from build123d import *

# Parameters (mm, degrees)
SKETCH_1_R           = 82.5
EXTRUDE_1_DEPTH      = 22.5
EXTRUDE_1_DEPTH_BACK = 22.5
SKETCH_4_R           = 67.5
CUT_EXTRUDE_1_DEPTH  = 4
SKETCH_5_R           = 52
CUT_EXTRUDE_2_DEPTH  = 48
CUT_EXTRUDE_3_DEPTH  = 2


with BuildPart() as part:
    # Sketch 1 → Extrude 1 (new body, two sides)
    with BuildSketch(Plane.XY) as extrude_1_sk:
        Circle(SKETCH_1_R)
    extrude(amount=EXTRUDE_1_DEPTH)
    extrude(extrude_1_sk.sketch, amount=-EXTRUDE_1_DEPTH_BACK)

    # Sketch 3 → Revolve 1 (revolve)
    with BuildSketch(Plane(origin=(0, 0, 0), x_dir=(0, 0, -1), z_dir=(1, 0, 0))):
        Polygon((-22.5, 0), (-22.5, 59.75), (-34.5, 52.75), (-34.5, 0), align=None)
    revolve(axis=Axis((0, 0, -22.110804518), (0, 0, 1)))

    # Sketch 4 → Cut-Extrude 1 (cut)
    with BuildSketch(Plane(origin=(0, 0, -22.5), x_dir=(-1, 0, 0), z_dir=(0, 0, -1))):
        Circle(SKETCH_4_R)
    extrude(amount=-CUT_EXTRUDE_1_DEPTH, mode=Mode.SUBTRACT)

    # Sketch 5 → Cut-Extrude 2 (cut)
    with BuildSketch(Plane(origin=(0, 0, -18.5), x_dir=(-1, 0, 0), z_dir=(0, 0, -1))):
        Circle(SKETCH_5_R)
    extrude(amount=-CUT_EXTRUDE_2_DEPTH, mode=Mode.SUBTRACT)

    # Sketch 7 → Cut-Revolve 1 (revolve, cut)
    with BuildSketch(Plane(origin=(0, 0, 0), x_dir=(0, 0, -1), z_dir=(1, 0, 0))):
        with BuildLine():
            Line((-22.5, 72.5), (-31.948658462, 72.5))
            Line((-31.948658462, 72.5), (-31.948658462, 102.607455118))
            Line((-31.948658462, 102.607455118), (33.489916399, 102.607455118))
            Line((33.489916399, 102.607455118), (33.489916399, 72.5))
            Line((33.489916399, 72.5), (22.5, 72.5))
            ThreePointArc((22.5, 72.5), (0, 79.75), (-22.5, 72.5))
        make_face()
    revolve(axis=Axis((0, 0, 0), (0, 0, 1)), mode=Mode.SUBTRACT)

    # Sketch 8 → Cut-Extrude 3 (cut)
    with BuildSketch(Plane.XY.offset(34.5)):
        with BuildLine():
            Line((-27.080041081, 26.318414926), (0, 28.434043135))
            Line((0, 28.434043135), (27.080041081, 26.318414926))
            Line((27.080041081, 26.318414926), (27.080041081, -1.78158165))
            ThreePointArc((27.080041081, -1.78158165), (17.912944533, -22.517713966), (0, -36.415528927))
            ThreePointArc((0, -36.415528927), (-17.912944533, -22.517713966), (-27.080041081, -1.78158165))
            Line((-27.080041081, -1.78158165), (-27.080041081, 26.318414926))
        make_face()
    extrude(amount=-CUT_EXTRUDE_3_DEPTH, mode=Mode.SUBTRACT)


solid = part.part
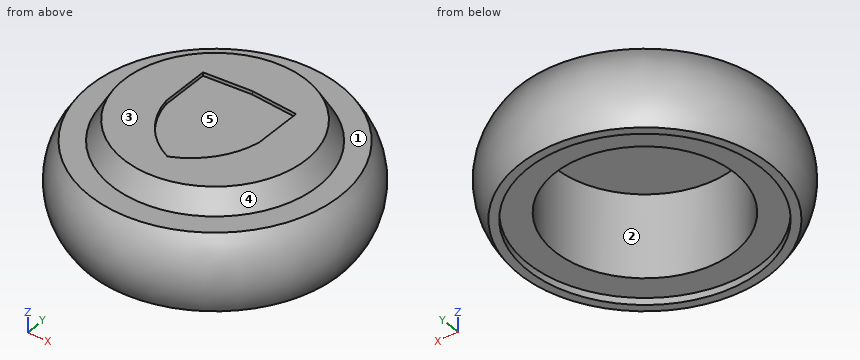
Read the model definition and answer for the solid it produces. Units are mm, in the model's axes. Face numbers are marked on the shaded views. A direction names the side the tool comes from. Coordinates: 2 decimals unless noted, no trailing zeros. Order: outer loops, then holes, each group sorted by start corner. A loop starts at its lowest first (then second) coordinate and runs counter-clockwise, first axis right, second up. Notation, with made-up numbers: M 59.25,-29 L 73.25,-29 A9 cw 73.25,-14 Z; hole C 5.5,1 d8. An arc over 180 degrees is marked long. Put each result on its own line as item: value. Start each with the question number.
Item 1: Section B-B, the plane z = -9 is taken. Determine the outline of the cut face in (x, y), plus the area to 3 significant figures.
Item 2: Consider probe 1 along Z at (x, y) = (29.5, -22.5); probe 2 along Y at (x, z) = (0, -19); probe 3 along Y at (x, z) = (0, -20.8). Determine where each line is inside the solid, lowest interval first. Write a range as [from, to].
Item 3: Section A-A, the plane z = 25.5 is taken. Determine the outline of the cut face in (x, y).
Item 4: The mould has two halves that part along Y. Classify the marked faces 3, 4 and 5: +Y half, -Y half, draft (parallel to the pull), parting line (faces both ways), or undercut.
Item 5: Given pin 1 Ø4 at (y, z) = (-47.5, -10) entering from +X; pin 2 Ø1.6 at (y, z) = (19, 33) entering from +X; pin 3 Ø12 at (y, z) = (-52, 14) entering from -X, each flat-ended and moving along its own axis, determine where each tip first touches the part or whether it passes through.
Item 6: For the marked faces 1 and 2, determine the directions among +Z, -Z, +X, -X, +Y, -Y from which every point of the face is accessible in a straight line to the end or side of a thin tool.
Computed:
1. outline: C 0,0 d157.37; hole C 0,0 d104
1. area: 11,000 mm2
2. probe 1: z = [29.5, 34.5]
2. probe 2: y = [-74.74, -67.5], [67.5, 74.74]
2. probe 3: y = [-73.65, -67.5], [67.5, 73.65]
3. outline: C 0,0 d116; hole C 0,0 d104
4. face 3: draft
4. face 4: parting line
4. face 5: undercut
5. pin 1: stops at x = 64.02
5. pin 2: stops at x = 50.73
5. pin 3: stops at x = -62.59
6. face 1: +Z
6. face 2: -Z
